Can you work these out from the model? Positions are in its coordinate system, mm. Face numbers are marked on the shaded views. A direction names the side the tool comes from. Coordinates: 2 decimals unless noted, no trailing zeros. Order: outer loops, then holes, each group sorted by start corner. A loop starts at its lowest first (then second) coordinate and runs counter-clockwise, first axis right, second up. Notation, with made-up numbers: (43.5, -31.75) - (86.5, -31.75) arc R18 cw to (86.5, 0.25) - close; hole circle Ø6 at (40.5, 41). An arc over 180 degrees is marked (long way). Return JSON: item names as keys, results as strings. Group by question number.
1) Imagine slicing it at B-B (z = 644). Write out the boundary of the cut face in (x, y), and give its area (3 significant figures).
2) For pin 1 Ø5 at (x, z) = (237.5, 500.5) entering from +Y; pin 2 Ø12 at (x, z) = (318.5, 769.5) entering from -Y; pin 3 Ø8 at (y, z) = (-108.5, 154) entering from +X, each with a flat end and sliding along its axis, tell me the tip position at first contact or that it passes through.
3) Imagine slicing it at A-A (z = 933). Write out the boundary of the cut face in (x, y), and give its area (3 significant figures).
4) If I drill on line 1 along Z through (x, y) = (432.5, -432); line 2 along X through (y, z) = (-197, 625.5); line 3 along X through (y, z) = (-285, 710), over which ranges is the centre line in solid material (lowest first)?
5) Which directions (+Z, -Z, +X, -X, +Y, -Y) give clear straight access to the entire face, cutting with the end or side of a thin tool? Please do the marked faces 1 and 2.
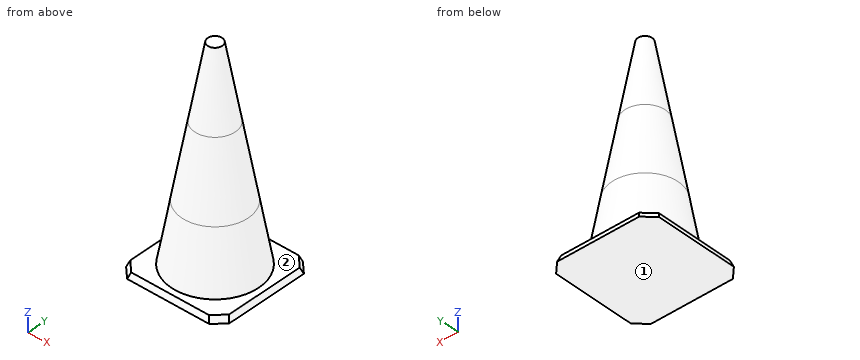
```python
from build123d import *

# Parameters (mm, degrees)
SKETCH_W     = 520
SKETCH_H     = 520
PAD_DEPTH    = 30
PAD_TAPER    = 20
CHAMFER_SIZE = 50
SKETCH001_R  = 220
PAD001_DEPTH = 300
PAD001_TAPER = 10
SKETCH002_R  = 167.101906
PAD002_DEPTH = 370
PAD002_TAPER = 10
SKETCH003_R  = 101.860923
PAD003_DEPTH = 370
PAD003_TAPER = 10


with BuildPart() as part:
    # Sketch → Pad (new body)
    with BuildSketch(Plane.XY):
        with Locations((260, -260)):
            Rectangle(SKETCH_W, SKETCH_H)
    extrude(amount=PAD_DEPTH, taper=PAD_TAPER)

    # Chamfer
    chamfer_edges = [part.edges().sort_by_distance(p)[0] for p in [
        (514.540446, -514.540446, 15),
        (514.540446, -5.459554, 15),
        (5.459554, -514.540446, 15),
        (5.459554, -5.459554, 15),
    ]]
    chamfer(chamfer_edges, length=CHAMFER_SIZE)

    # Sketch001 (on Face5 of Chamfer) → Pad001 (join)
    with BuildSketch(Plane.XY.offset(30)):
        with Locations((260, -260)):
            Circle(SKETCH001_R)
    extrude(amount=PAD001_DEPTH, taper=PAD001_TAPER)

    # Sketch002 (on Face12 of Pad001) → Pad002 (join)
    with BuildSketch(Plane.XY.offset(330)):
        with Locations((260, -260)):
            Circle(SKETCH002_R)
    extrude(amount=PAD002_DEPTH, taper=PAD002_TAPER)

    # Sketch003 (on Face13 of Pad002) → Pad003 (join)
    with BuildSketch(Plane.XY.offset(700)):
        with Locations((260, -260)):
            Circle(SKETCH003_R)
    extrude(amount=PAD003_DEPTH, taper=PAD003_TAPER)


solid = part.part
```
Calculated:
{
 "1": {"outline": "circle Ø223.47 at (260, -260)", "area": "39,200 mm2"},
 "2": {"pin 1": "y = -124.22", "pin 2": "y = -332.81", "pin 3": "x = 392.42"},
 "3": {"outline": "circle Ø121.55 at (260, -260)", "area": "11,600 mm2"},
 "4": {"line 1": "0 to 30", "line 2": "163.8 to 356.2", "line 3": "163.07 to 356.93"},
 "5": {"face 1": "-Z, +X, -X, +Y, -Y", "face 2": "+Z"}
}
